```python
from build123d import *

# Parameters (mm, degrees)
F0_W     = 3
F0_H     = 30
F0_W_2   = 114
F1_DEPTH = 3
F2_DEPTH = 28
F0_W_3   = 15
F0_R     = 1.75
F3_DEPTH = 3
F4_R     = 1.75
F5_DEPTH = 200


with BuildPart() as f1:
    # F0 (on Top) → F1 (new body)
    with BuildSketch(Plane.XY):
        with Locations((-1.5, 15)):
            Rectangle(F0_W, F0_H)
        with Locations((57, 15)):
            Rectangle(F0_W_2, F0_H)
        with Locations((115.5, 15)):
            Rectangle(F0_W, F0_H)
    extrude(amount=-F1_DEPTH)

    # F0 (on Top) → F2 (join)
    with BuildSketch(Plane.XY):
        with Locations((-1.5, 15)):
            Rectangle(F0_W, F0_H)
        with Locations((115.5, 15)):
            Rectangle(F0_W, F0_H)
    extrude(amount=F2_DEPTH)

    # F0 (on Top) → F3 (join)
    with BuildSketch(Plane.XY):
        with Locations((-10.5, 15)):
            Rectangle(F0_W_3, F0_H)
        with Locations((-10.5, 15)):
            Circle(F0_R, mode=Mode.SUBTRACT)
        with Locations((124.5, 15)):
            Rectangle(F0_W_3, F0_H)
        with Locations((124.5, 15)):
            Circle(F0_R, mode=Mode.SUBTRACT)
    extrude(amount=-F3_DEPTH)

    # F4 (on face) → F5 (cut)
    with BuildSketch(Plane.YZ.offset(117)):
        with Locations((15, 11.299537)):
            Circle(F4_R)
    extrude(amount=-F5_DEPTH, mode=Mode.SUBTRACT)


solid = f1.part
```
Check sheet for the modelled part. Datum: model origin and axes. Units: mm. A direction names the side the tool comes from. Give positions to 0.01 mm unless a question says otherwise; leave off trailing zeros. Write each loop counter-clockwise with the first axis right and the second up, starting at its lowest first coordinate (ties: lowest second). Pieces come first, ordered by that corner, then holes. Notation, with made-up numbers: (4, 40.25) - (23, 40.25) arc R24 ccw to (23, 71.25) - close; hole circle Ø9 at (83.25, 40). An arc over 180 degrees is marked (long way). Answer as a JSON object with one key per item and string values. Group by question number.
1) Depth check by flat-ended pin: P1, Ø8.5, axis at y = 8.5, z = 12, coming from the -X side; P2, Ø3, axis at y = 15, z = 11.3, coming from the +X side; P3, Ø4, axis at x = -10.5, y = 15, coming from the -Z side; P4, Ø12, axis at x = 124.5, y = 12, coming from the +Z side. Enter the tip coordinate at first touch or a pass-through.
2) Thickness scan on probe 1 along X at (y, z) = (20.5, 2); probe 2 along Y at (x, z) = (-10.5, -1.75); probe 3 along Z at (x, y) = (28, 7). Record the ranges inside material, lowest first. Write a range as from..to.
3) Release check for a two-part mould opening along Y. For faces 4 (the face through (57, 30, -1)), 5 (the face through (-10.728, 16.735, -1.479)), 6 (the face through (115.521, 16.669, 11.825)), 7 (the face through (56, 15, -3)) record: pulls with the +Y half, pulls with the -Y half, needs draft (parallel to the pull), parting line crosses it, or undercut.
4) Sectioned sample at A-A (z = 6). Record the cut outline in (x, y), then the cut area to 3 significant figures.
5) Sectioned sample at B-B (x = -10.5). Record the cut outline in (y, z), then the cut area to 3 significant figures.
6) Sectioned sample at D-D (y = 25). Record the cut outline in (x, z).
7) Access from +Z, -Z, +X, -X, +Y, -Y to the whole of each face (thin tool, end or side, straight path). Record for faces 1 (the face through (0, 15, 14)), 2 (the face through (-14, 15, 0)), 3 (the face through (121, 15, 0)).
8) Sectioned sample at C-C (y = 15). Record the cut outline in (x, z).
Geometry results:
{
 "1": {"P1": "stops at x = -3", "P2": "passes through", "P3": "stops at z = -3", "P4": "stops at z = 0"},
 "2": {"probe 1": "x = -3..0, 114..117", "probe 2": "y = 0..13.25, 16.75..30", "probe 3": "z = -3..0"},
 "3": {"face 4": "pulls with the +Y half", "face 5": "undercut", "face 6": "undercut", "face 7": "needs draft"},
 "4": {"outline": "(-3, 0) - (0, 0) - (0, 30) - (-3, 30) - close; (114, 0) - (117, 0) - (117, 30) - (114, 30) - close", "area": "180 mm^2"},
 "5": {"outline": "(0, -3) - (13.25, -3) - (13.25, 0) - (0, 0) - close; (16.75, -3) - (30, -3) - (30, 0) - (16.75, 0) - close", "area": "79.5 mm^2"},
 "6": {"outline": "(-18, -3) - (132, -3) - (132, 0) - (117, 0) - (117, 28) - (114, 28) - (114, 0) - (0, 0) - (0, 28) - (-3, 28) - (-3, 0) - (-18, 0) - close"},
 "7": {"face 1": "+Z, +Y, -Y", "face 2": "+Z, -X, +Y, -Y", "face 3": "+Z, +X, +Y, -Y"},
 "8": {"outline": "(-18, -3) - (-12.25, -3) - (-12.25, 0) - (-18, 0) - close; (-8.75, -3) - (122.75, -3) - (122.75, 0) - (117, 0) - (117, 9.55) - (114, 9.55) - (114, 0) - (0, 0) - (0, 9.55) - (-3, 9.55) - (-3, 0) - (-8.75, 0) - close; (-3, 13.05) - (0, 13.05) - (0, 28) - (-3, 28) - close; (114, 13.05) - (117, 13.05) - (117, 28) - (114, 28) - close; (126.25, -3) - (132, -3) - (132, 0) - (126.25, 0) - close"}
}
